```python
from build123d import *

# Parameters (mm, degrees)
BOSS_EXTRUDE1_DEPTH = 6.35
SKETCH4_W           = 10.16
SKETCH4_H           = 28.575
BOSS_EXTRUDE4_DEPTH = 101.6
SKETCH5_W           = 10.16
SKETCH5_H           = 28.575
BOSS_EXTRUDE5_DEPTH = 101.6
SKETCH6_W           = 10.16
SKETCH6_H           = 25.4
BOSS_EXTRUDE7_DEPTH = 101.6
FILLET2_R           = 5.08
FILLET3_R           = 5.08
FILLET4_R           = 5.08
FILLET5_R           = 5.08
FILLET6_R           = 5.08
FILLET7_R           = 5.08
FILLET8_R           = 2.54
FILLET9_R           = 2.54


with BuildPart() as part:
    # Sketch1 → Boss-Extrude1 (new body)
    with BuildSketch(Plane(origin=(0, 0, 0), x_dir=(1, 0, 0), z_dir=(0, 1, 0))):
        Polygon((0, 114.3), (0, 139.7), (-95.25, 139.7), (-95.25, 111.125), (-25.4, 111.125), (-25.4, 3.175), (-95.25, 3.175), (-95.25, -25.4), (0, -25.4), (0, 0), (69.85, 0), (69.85, 114.3), align=None)
    extrude(amount=BOSS_EXTRUDE1_DEPTH)

    # Sketch4 → Boss-Extrude4 (add)
    with BuildSketch(Plane(origin=(0, 6.35, 0), x_dir=(1, 0, 0), z_dir=(0, 1, 0))):
        with Locations((-90.17, -11.1125)):
            Rectangle(SKETCH4_W, SKETCH4_H)
        with Locations((-46.99, -11.1125)):
            Rectangle(SKETCH4_W, SKETCH4_H)
    extrude(amount=BOSS_EXTRUDE4_DEPTH)

    # Sketch5 → Boss-Extrude5 (add)
    with BuildSketch(Plane(origin=(0, 6.35, 0), x_dir=(1, 0, 0), z_dir=(0, 1, 0))):
        with Locations((-90.17, 125.4125)):
            Rectangle(SKETCH5_W, SKETCH5_H)
        with Locations((-46.99, 125.4125)):
            Rectangle(SKETCH5_W, SKETCH5_H)
    extrude(amount=BOSS_EXTRUDE5_DEPTH)

    # Sketch6 → Boss-Extrude7 (add)
    with BuildSketch(Plane(origin=(0, 6.35, 0), x_dir=(1, 0, 0), z_dir=(0, 1, 0))):
        with Locations((64.77, 57.15)):
            Rectangle(SKETCH6_W, SKETCH6_H)
    extrude(amount=BOSS_EXTRUDE7_DEPTH)

    # Fillet2
    fillet2_edges = [part.edges().sort_by_distance(p)[0] for p in [
        (-41.91, 6.35, 11.1125),
    ]]
    fillet(fillet2_edges, radius=FILLET2_R)

    # Fillet3
    fillet3_edges = [part.edges().sort_by_distance(p)[0] for p in [
        (-52.07, 6.35, 11.1125),
    ]]
    fillet(fillet3_edges, radius=FILLET3_R)

    # Fillet4
    fillet4_edges = [part.edges().sort_by_distance(p)[0] for p in [
        (-85.09, 6.35, 11.1125),
    ]]
    fillet(fillet4_edges, radius=FILLET4_R)

    # Fillet5
    fillet5_edges = [part.edges().sort_by_distance(p)[0] for p in [
        (-85.09, 6.35, -125.4125),
    ]]
    fillet(fillet5_edges, radius=FILLET5_R)

    # Fillet6
    fillet6_edges = [part.edges().sort_by_distance(p)[0] for p in [
        (-52.07, 6.35, -125.4125),
    ]]
    fillet(fillet6_edges, radius=FILLET6_R)

    # Fillet7
    fillet7_edges = [part.edges().sort_by_distance(p)[0] for p in [
        (-41.91, 6.35, -125.4125),
    ]]
    fillet(fillet7_edges, radius=FILLET7_R)

    # Fillet8
    fillet8_edges = [part.edges().sort_by_distance(p)[0] for p in [
        (64.77, 6.35, -44.45),
    ]]
    fillet(fillet8_edges, radius=FILLET8_R)

    # Fillet9
    fillet9_edges = [part.edges().sort_by_distance(p)[0] for p in [
        (64.77, 6.35, -69.85),
    ]]
    fillet(fillet9_edges, radius=FILLET9_R)


solid = part.part
```
Work out the finished part from the listing and answer in its coordinate system (mm). A direction names the side the tool comes from. Give positions to 0.01 mm unless a question says otherwise; leave off trailing zeros. Write each loop counter-clockwise with the first axis right and the second up, starting at its lowest first coordinate (ties: lowest second). Pieces come first, ordered by that corner, then holes.
(1) The part is cut by section B-B on y = 21. Write down the section's boundary in (x, z) (3 decimals).
Final values:
outline: (-95.25, -139.7) - (-85.09, -139.7) - (-85.09, -111.125) - (-95.25, -111.125) - close; (-95.25, -3.175) - (-85.09, -3.175) - (-85.09, 25.4) - (-95.25, 25.4) - close; (-52.07, -139.7) - (-41.91, -139.7) - (-41.91, -111.125) - (-52.07, -111.125) - close; (-52.07, -3.175) - (-41.91, -3.175) - (-41.91, 25.4) - (-52.07, 25.4) - close; (59.69, -69.85) - (69.85, -69.85) - (69.85, -44.45) - (59.69, -44.45) - close
(2) Which of the six approach directions +Z, -Z, +X, -X, +Y, -Y give full straight-line access (tool end or side, diameter ignored) to faces 4 (the flat face through (0, 3, 13)), 5 (the flat face through (-50, 42, -3.175)), 6 (the flat face through (0, 3, -127)), 7 (the flat face through (-69, 6.35, -126)), 8 (the flat face through (-41.91, 59, 11))?
Final values:
face 4: +Z, +X, +Y, -Y
face 5: -X, +Y, -Y
face 6: -Z, +X, +Y, -Y
face 7: +Z, -Z, +Y
face 8: +Z, -Z, +X, +Y
(3) The part is cut by section C-C on z = -79. Write down the section's boundary in (x, y).
Final values:
outline: (-25.4, 0) - (69.85, 0) - (69.85, 6.35) - (-25.4, 6.35) - close
(4) The mould has two halves that part along Z. Classify faces 1 (the flat face through (-85.09, 59, 11)), 2 (the flat face through (-51, 46, 25.4)), 3 (the flat face through (-25.4, 3, -58)): pulls with the +Z half, pulls with the -Z half, needs draft (parallel to the pull), parting line crosses it, or undercut.
Final values:
face 1: needs draft
face 2: pulls with the +Z half
face 3: undercut
(5) Flat-ended cylindrical pins translate along their axes: pin 1 Ø6 at (y, z) = (21.5, -5) entering from +X; pin 2 Ø18.5 at (x, z) = (-70, 12.5) entering from +Y; pin 3 Ø21 at (x, y) = (-71, 76.5) entering from +Z; pin 4 Ø8 at (x, y) = (65.5, 48) entering from +Z. Find the tip coordinate at first contact, or state that the pin passes through.
Final values:
pin 1: stops at x = -41.91
pin 2: stops at y = 6.35
pin 3: passes through
pin 4: stops at z = -44.45
(6) Straight lines are drawn through the part: line 1 (Z direction, x = -47, y = 66) (3 decimals); line 2 (X direction, y = 72, z = 6); line 3 (Z direction, x = 63.5, y = 31). For each, find the intervals that lie inside material, in ascending order.
Final values:
line 1: z = -139.7 to -111.125, -3.175 to 25.4
line 2: x = -95.25 to -85.09, -52.07 to -41.91
line 3: z = -69.85 to -44.45
(7) The part is cut by section D-D on x = 29.5. Write down the section's boundary in (y, z).
Final values:
outline: (0, -114.3) - (6.35, -114.3) - (6.35, 0) - (0, 0) - close
(8) The part is cut by section A-A on x = -77.5. Write down the section's boundary in (y, z) (3 decimals), plus the area to 3 significant figures.
Final values:
outline: (0, -139.7) - (6.35, -139.7) - (6.35, -111.125) - (0, -111.125) - close; (0, -3.175) - (6.35, -3.175) - (6.35, 25.4) - (0, 25.4) - close
area: 363 mm2
